Can you work these out from the model? Positions are in its coordinate system, mm. A direction names the side the tool comes from. Give positions to 0.01 mm unless a question says otherwise; leave off trailing zeros. Loops run counter-clockwise (first coordinate to the right, second up) from the corner with the lowest first, then second, coordinate; pieces in that order, holes last. Notation, with made-up numbers: (-11.75, -23.75) - (34.25, -23.75) arc R25 cw to (34.25, 15.25) - close; hole circle Ø6 at (-31.5, 71.25). An arc over 180 degrees is marked (long way). Use a Markdown table: item, result. Add a question column.
```python
from build123d import *

# Parameters (mm, degrees)
BOSS_EXTRUDE1_DEPTH = 286.639
SKETCH2_R           = 2.4892
CUT_EXTRUDE1_DEPTH  = 25.4
SKETCH3_R           = 2.4892
CUT_EXTRUDE2_DEPTH  = 25.4


with BuildPart() as part:
    # Sketch1 → Boss-Extrude1 (new body)
    with BuildSketch(Plane(origin=(0, 0, 0), x_dir=(1, 0, 0), z_dir=(0, 1, 0))):
        Polygon((0, 7.332348419), (-6.35, 3.666174209), (-6.35, -3.666174209), (0, -7.332348419), (6.35, -3.666174209), (6.35, 3.666174209), align=None)
    extrude(amount=BOSS_EXTRUDE1_DEPTH)

    # Sketch2 → Cut-Extrude1 (cut)
    with BuildSketch(Plane(origin=(0, 286.639, 0), x_dir=(1, 0, 0), z_dir=(0, 1, 0))):
        Circle(SKETCH2_R)
    extrude(amount=-CUT_EXTRUDE1_DEPTH, mode=Mode.SUBTRACT)

    # Sketch3 → Cut-Extrude2 (cut)
    with BuildSketch(Plane(origin=(0, 0, 0), x_dir=(-1, 0, 0), z_dir=(0, -1, 0))):
        Circle(SKETCH3_R)
    extrude(amount=-CUT_EXTRUDE2_DEPTH, mode=Mode.SUBTRACT)


solid = part.part
```
1. Will these pins go through, and if not, where does the flat tip stop? P1, Ø5, axis at x = 1, y = 162, coming from the -Z side; P2, Ø1, axis at x = -3, y = 70, coming from the -Z side; P3, Ø2.5, axis at x = 0.5, z = 1, coming from the +Y side.
2. On a 3-axis mill with a long thin cutter (end or side, diameter ignored), from which of +Z, -Z, +X, -X, +Y, -Y can I reach the whole of each face in a straight line? I mean faces 1 (the face through (0, 261.239, 0)), 2 (the face through (3.219, 141.313, -5.474)), 3 (the face through (0, 25.4, 0)). Say none if no direction works.
3. If we mould it in two halves opening along X, with no side actions, what happens to faces 4 (the face through (2.374, 274.117, -0.748)), 5 (the face through (0, 286.639, 3)), 6 (the face through (6.35, 141, 0))? For each: released by +X, released by -X, zero draft, split by the parting line, or undercut.
4. Suppose I cut it at B-B (y = 81.5). List the corners of the cut face in (x, z) for me.
5. Please list where these lines run through material, in increasing order: line 1 along X through (y, z) = (277.75, 0); line 2 along Z through (x, y) = (0, 270.5); line 3 along Y through (x, z) = (-1, -1.25). Write a range as [from, to].
6. Suppose I cut it at A-A (z = 0). List the corners of the cut face in (x, y) for me.
Results below:
| question | item | result |
|---|---|---|
| 1 | P1 | z = -7.33 |
| 1 | P2 | z = -5.89 |
| 1 | P3 | y = 261.24 |
| 2 | face 1 | +Y |
| 2 | face 2 | -Z, +X, +Y, -Y |
| 2 | face 3 | -Y |
| 3 | face 4 | undercut |
| 3 | face 5 | zero draft |
| 3 | face 6 | released by +X |
| 4 | outline | (-6.35, -3.67) - (0, -7.33) - (6.35, -3.67) - (6.35, 3.67) - (0, 7.33) - (-6.35, 3.67) - close |
| 5 | line 1 | [-6.35, -2.49], [2.49, 6.35] |
| 5 | line 2 | [-7.33, -2.49], [2.49, 7.33] |
| 5 | line 3 | [25.4, 261.24] |
| 6 | outline | (-6.35, 0) - (-2.49, 0) - (-2.49, 25.4) - (2.49, 25.4) - (2.49, 0) - (6.35, 0) - (6.35, 286.64) - (2.49, 286.64) - (2.49, 261.24) - (-2.49, 261.24) - (-2.49, 286.64) - (-6.35, 286.64) - close |
